```python
from build123d import *

# Parameters (mm, degrees)
TOP_PLATE_BOSS_EXTRUDE1_DEPTH                  = 25
TOP_PLATE_BOSS_EXTRUDE1_DEPTH_BACK             = 25
SKETCH5_R                                      = 5
SHAFT_CUT_EXTRUDE1_DEPTH                       = 8
SKETCH6_R                                      = 8
SHAFT_BEARING_CUT_EXTRUDE2_DEPTH               = 2.5
SKETCH7_R                                      = 1.5
BEARING_PLATE_MOUNTING_HOLES_CUT_EXTRUDE_DEPTH = 8
SKETCH8_R                                      = 1.5
BASE_SIDE_MOUNTING_HOLES_CUT_EXTRUDE4_DEPTH    = 8
SKETCH9_W                                      = 53
SKETCH9_H                                      = 40
TIMING_BELT_SLIDER_HOLE_CUT_EXTRUDE1_DEPTH     = 8


with BuildPart() as part:
    # Sketch2 → Top Plate Boss-Extrude1 (new, two sides: drawn at the far end of the back side and taken through both)
    with BuildSketch(Plane.XY.offset(-TOP_PLATE_BOSS_EXTRUDE1_DEPTH_BACK)):
        Polygon((-86.592068141, 50), (86.592068141, 50), (87.404678508, 42), (-87.404678508, 42), align=None)
    extrude(amount=TOP_PLATE_BOSS_EXTRUDE1_DEPTH + TOP_PLATE_BOSS_EXTRUDE1_DEPTH_BACK)

    # Sketch4 → Top Plate Chassi Rounding Cut-Revolve1 (revolve, cut)
    with BuildSketch(Plane.XY):
        Polygon((86.592068141, 50), (87.404678508, 42), (97.784973569, 42), (97.784973569, 50), align=None)
    revolve(axis=Axis((0, 0, 0), (0, 1, 0)), mode=Mode.SUBTRACT)

    # Sketch5 → Shaft Cut-Extrude1 (cut)
    with BuildSketch(Plane.XZ.offset(-42)):
        Circle(SKETCH5_R)
    extrude(amount=-SHAFT_CUT_EXTRUDE1_DEPTH, mode=Mode.SUBTRACT)

    # Sketch6 → Shaft Bearing Cut-Extrude2 (cut)
    with BuildSketch(Plane.XZ.offset(-42)):
        Circle(SKETCH6_R)
    extrude(amount=-SHAFT_BEARING_CUT_EXTRUDE2_DEPTH, mode=Mode.SUBTRACT)

    # Sketch7 → Bearing Plate Mounting Holes Cut-Extrude3 (cut)
    with BuildSketch(Plane.XZ.offset(-42)):
        with Locations((12, 20)):
            Circle(SKETCH7_R)
        with Locations((-12, 20)):
            Circle(SKETCH7_R)
        with Locations((-12, -20)):
            Circle(SKETCH7_R)
        with Locations((12, -20)):
            Circle(SKETCH7_R)
    extrude(amount=-BEARING_PLATE_MOUNTING_HOLES_CUT_EXTRUDE_DEPTH, mode=Mode.SUBTRACT)

    # Sketch8 → Base Side Mounting Holes Cut-Extrude4 (cut)
    with BuildSketch(Plane.XZ.offset(-42)):
        with Locations((21, 20)):
            Circle(SKETCH8_R)
        with Locations((-21, 20)):
            Circle(SKETCH8_R)
        with Locations((-21, -20)):
            Circle(SKETCH8_R)
        with Locations((21, -20)):
            Circle(SKETCH8_R)
    extrude(amount=-BASE_SIDE_MOUNTING_HOLES_CUT_EXTRUDE4_DEPTH, mode=Mode.SUBTRACT)

    # Sketch9 → Timing Belt Slider Hole Cut-Extrude1 (cut)
    with BuildSketch(Plane(origin=(0, 50, 0), x_dir=(1, 0, 0), z_dir=(0, 1, 0))):
        with Locations((55.5, 0)):
            Rectangle(SKETCH9_W, SKETCH9_H)
    extrude(amount=-TIMING_BELT_SLIDER_HOLE_CUT_EXTRUDE1_DEPTH, mode=Mode.SUBTRACT)


solid = part.part
```
CAD build for the part. Positions are in the model's coordinates, mm. A direction names the side the tool comes from. Round coordinates to 2 decimals unless told otherwise and drop trailing zeros. Write each loop counter-clockwise with the first axis right and the second up, starting at its lowest first coordinate (ties: lowest second). Pieces come first, ordered by that corner, then holes. Notation, with made-up numbers: (29.25, 16.5) - (61.25, 16.5) arc R26 cw to (61.25, 44.5) - close; hole circle Ø1 at (-28.5, -5). An arc over 180 degrees is marked (long way). Write item = value, one per line. Start each with the question number.
Q1. Band-saw the part on A-A (x = 21). Give the cut face in (y, z), then the cut area to 3 significant figures.
Q2. Band-saw the part on C-C (y = 48). Count the separate pieces of the cut face and the enclosed holes in it, then the cut area to 3 significant figures.
Q3. Band-saw the part on B-B (x = 0). Give the cut face in (y, z).
Q4. Which spindle directions (+Z, -Z, +X, -X, +Y, -Y) get a long thin tool onto all of the face, cutting with end or side? Do faces 5 (the flat face through (55, 46, -20)), 6 (the conical face through (-87, 46, 0)), 7 (the cylindrical face through (-1.73, 43.23, -7.81)). Say none if no direction does.
Q5. Mould opens along Z. For faces 1 (the flat face through (82, 46, 0)), 2 (the flat face through (1, 46, -25)), 3 (the flat face through (-18, 42, 0)), 4 (the cylindrical face through (-22.11, 45.94, 21.01)) say: pulls with the +Z half, pulls with the -Z half, needs draft (parallel to the pull), parting line crosses it, or undercut.
Q6. Probe L1, parallel to Z at x = -21, y = 47.75; L2, parallel to Z at x = 50, y = 46.5; L3, parallel to X at y = 46.75, z = -1.5. List the from-to ranges inside material, lowest first. Write a range as from..to.
Q7. Drop flat-ended pins along their axis: pin 1 (3 mm diameter, centred on y = 48, z = -10.5, fed in from +X); pin 2 (2.5 mm diameter, centred on y = 47, z = -5.5, fed in from +X); pin 3 (3 mm diameter, centred on y = 48, z = -11, fed in from +X). Give the stop position or say it passes through.
Answers below:
q1.outline = (42, -25) - (50, -25) - (50, -21.5) - (42, -21.5) - close; (42, -18.5) - (50, -18.5) - (50, 18.5) - (42, 18.5) - close; (42, 21.5) - (50, 21.5) - (50, 25) - (42, 25) - close
q1.area = 352 mm2
q2.separate_pieces = 1
q2.enclosed_holes = 10
q2.area = 6,300 mm2
q3.outline = (42, -25) - (50, -25) - (50, -5) - (44.5, -5) - (44.5, -8) - (42, -8) - close; (42, 8) - (44.5, 8) - (44.5, 5) - (50, 5) - (50, 25) - (42, 25) - close
q4.face_5 = +Y, -Y
q4.face_6 = -X, +Y
q4.face_7 = -Y
q5.face_1 = undercut
q5.face_2 = pulls with the -Z half
q5.face_3 = needs draft
q5.face_4 = undercut
q6.L1 = -25..-21.5, -18.5..18.5, 21.5..25
q6.L2 = -25..-20, 20..25
q6.L3 = -86.91..-4.77, 4.77..29, 82..86.91
q7.pin_1 = 86.39
q7.pin_2 = 86.87
q7.pin_3 = 86.33
